Check sheet for the modelled part. Datum: model origin and axes. Units: mm. A direction names the side the tool comes from. Round coordinates to 2 decimals unless told otherwise and drop trailing zeros. Write each loop counter-clockwise with the first axis right and the second up, starting at its lowest first coordinate (ties: lowest second). Pieces come first, ordered by that corner, then holes. Notation, with made-up numbers: (59.25, -36) -> (106.25, -36) arc R27 cw to (106.25, -1) -> close; hole circle Ø2 at (19, -31.5). An arc over 180 degrees is marked (long way). Write item = value, one per line.
from build123d import *

# Parameters (mm, degrees)
F1_R     = 30
F2_DEPTH = 10
F5_DEPTH = 40
F3_R     = 30
F3_R_2   = 27.5
F6_DEPTH = 20


with BuildPart() as f2:
    # F1 (on face) → F2 (new body)
    with BuildSketch(Plane.XY):
        Circle(F1_R)
        with BuildLine():
            ThreePointArc((2.6, 0), (-1.8887723072, -1.7867678001), (0.1442006372, 2.5959981079))
            Line((0.1442006372, 2.5959981079), (1.3613009588, 1.465216605))
            Line((1.3613009588, 1.465216605), (2.5784012803, 0.3344351021))
            ThreePointArc((2.5784012803, 0.3344351021), (2.5945947014, 0.1675659141), (2.6, 0))
        make_face(mode=Mode.SUBTRACT)
    extrude(amount=F2_DEPTH)

    # F4 (on face) → F5 (join)
    with BuildSketch(Plane(origin=(0, 0, 0), x_dir=(1, 0, 0), z_dir=(0, 0, -1))):
        with BuildLine():
            Line((25.6627975095, 9.8828550524), (21.2857162159, 5.5604213128))
            Line((21.2857162159, 5.5604213128), (27.2175942873, 3.9309745879))
            ThreePointArc((27.2175942873, 3.9309745879), (26.6071452699, 6.950526641), (25.6627975095, 9.8828550524))
        make_face()
        with BuildLine():
            Line((21.390202292, -17.2832070492), (15.4583242206, -15.6537603243))
            Line((15.4583242206, -15.6537603243), (17.0131209984, -21.6056407888))
            ThreePointArc((17.0131209984, -21.6056407888), (19.3229052758, -19.5672004054), (21.390202292, -17.2832070492))
        make_face()
        with BuildLine():
            Line((4.2725952175, 27.1660621016), (5.8273919953, 21.2141816371))
            Line((5.8273919953, 21.2141816371), (10.2044732889, 25.5366153767))
            ThreePointArc((10.2044732889, 25.5366153767), (7.2842399941, 26.5177270464), (4.2725952175, 27.1660621016))
        make_face()
        with BuildLine():
            Line((-4.2725952175, -27.1660621016), (-5.8273919953, -21.2141816371))
            Line((-5.8273919953, -21.2141816371), (-10.2044732889, -25.5366153767))
            ThreePointArc((-10.2044732889, -25.5366153767), (-7.2842399941, -26.5177270464), (-4.2725952175, -27.1660621016))
        make_face()
        with BuildLine():
            Line((-21.390202292, 17.2832070492), (-15.4583242206, 15.6537603243))
            Line((-15.4583242206, 15.6537603243), (-17.0131209984, 21.6056407888))
            ThreePointArc((-17.0131209984, 21.6056407888), (-19.3229052758, 19.5672004054), (-21.390202292, 17.2832070492))
        make_face()
        with BuildLine():
            Line((-25.6627975095, -9.8828550524), (-21.2857162159, -5.5604213128))
            Line((-21.2857162159, -5.5604213128), (-27.2175942873, -3.9309745879))
            ThreePointArc((-27.2175942873, -3.9309745879), (-26.6071452699, -6.950526641), (-25.6627975095, -9.8828550524))
        make_face()
    extrude(amount=F5_DEPTH)

    # F3 (on face) → F6 (join)
    with BuildSketch(Plane(origin=(0, 0, 0), x_dir=(1, 0, 0), z_dir=(0, 0, -1))):
        Circle(F3_R)
        Circle(F3_R_2, mode=Mode.SUBTRACT)
    extrude(amount=F6_DEPTH)


solid = f2.part
(1) Go/stop test with flat-tipped pins: P1, Ø3, axis at x = 2, y = 3.5, coming from the -Z side; P2, Ø8, axis at x = 10, z = -1.5, coming from the -Y side; P3, Ø10, axis at x = 10.5, z = -3.5, coming from the +Y side. Record where each tip stops, or that it passes through.
Worked answers:
P1 = 0
P2 = -29.39
P3 = 29.49
(2) Sectioned sample at C-C on x = -7.5. Enter the section's corners in (y, z), then the cut area to 3 significant figures.
Worked answers:
outline = (-29.05, -20) -> (-26.46, -20) -> (-26.46, 0) -> (22.87, 0) -> (22.87, -40) -> (26.46, -40) -> (26.46, -20) -> (29.05, -20) -> (29.05, 10) -> (-29.05, 10) -> close
area = 828 mm²
(3) Release check for a two-part mould opening along X. For faces 1 (the cylindrical face through (7.326, -26.506, -29.86)), 2 (the flat face through (-18.47, -16.48, -19.72)), 3 (the flat face through (25, -6, -40)) record: pulls with the +X half, pulls with the -X half, needs draft (parallel to the pull), parting line crosses it, or undercut.
Worked answers:
face_1 = pulls with the +X half
face_2 = undercut
face_3 = needs draft
(4) Sectioned sample at D-D on z = 5. Enter the section's corners in (x, y), then the cut area to 3 significant figures.
Worked answers:
outline = circle Ø60 at (0, 0); hole (0.14, 2.6) arc R2.6 ccw (long way) to (2.58, 0.33) -> close
area = 2,810 mm²
(5) Access from +Z, -Z, +X, -X, +Y, -Y to the whole of each face (thin tool, end or side, straight path). Record for faces 4 (the flat face through (16.225, 18.588, -19.72)), 5 (the cylindrical face through (-29.97, -1.32, -4.79)).
Worked answers:
face_4 = -Z
face_5 = +Z, -Z
(6) Material ranges on L1, parallel to Y at x = 0, z = 6; L2, parallel to Z at x = -22, y = -2; L3, parallel to Y at x = -1, z = -18.5, recorded low to high. Write a range as [from, to].
Worked answers:
L1 = [-30, -2.6], [2.6, 30]
L2 = [0, 10]
L3 = [-29.98, -27.48], [27.48, 29.98]
(7) Sectioned sample at B-B on y = -11.5. Enter the section's corners in (x, z), then the cut area to 3 significant figures.
Worked answers:
outline = (-27.71, -20) -> (-24.98, -20) -> (-24.98, 0) -> (24.98, 0) -> (24.98, -20) -> (27.71, -20) -> (27.71, 10) -> (-27.71, 10) -> close
area = 663 mm²
(8) Sectioned sample at A-A on z = -24.5. Enter the section's corners in (x, y), then the cut area to 3 significant figures.
Worked answers:
outline = (-27.22, 3.93) -> (-21.29, 5.56) -> (-25.66, 9.88) arc R27.5 ccw to start; (-21.39, -17.28) arc R27.5 ccw to (-17.01, -21.61) -> (-15.46, -15.65) -> close; (-10.2, 25.54) -> (-5.83, 21.21) -> (-4.27, 27.17) arc R27.5 ccw to start; (4.27, -27.17) arc R27.5 ccw to (10.2, -25.54) -> (5.83, -21.21) -> close; (15.46, 15.65) -> (21.39, 17.28) arc R27.5 ccw to (17.01, 21.61) -> close; (21.29, -5.56) -> (25.66, -9.88) arc R27.5 ccw to (27.22, -3.93) -> close
area = 103 mm²
